Autodesk Fusion 360 part; units mm, degrees
sketch "Sketch1" plane through (0, 0, 0) normal (0, 0, 1) x (1, 0, 0)
  line L0 (0, 0) -> (385.5, 0)
  line L1 (385.5, 0) -> (385.5, 160.5)
  line L2 (385.5, 160.5) -> (0, 160.5)
  line L3 (0, 160.5) -> (0, 0)
  line L4 (10, 150.5) -> (375.5, 150.5)
  line L5 (375.5, 150.5) -> (375.5, 10)
  line L6 (375.5, 10) -> (10, 10)
  line L7 (10, 10) -> (10, 150.5)
  circle A0 centre (5, 155.5) radius 1.45
  circle A1 centre (5, 5) radius 1.45
  circle A2 centre (380.5, 5) radius 1.45
  circle A3 centre (380.5, 155.5) radius 1.45
  dimension "d1" = 160.5
  dimension "d2" = 385.5
  dimension "d3" = 10
  dimension "d4" = 10
  dimension "d5" = 10
  dimension "d6" = 10
  dimension "d7" = 2.9
  dimension "d8" = 2.9
  dimension "d9" = 2.9
  dimension "d10" = 2.9
  dimension "d11" = 5
  dimension "d12" = 5
  dimension "d13" = 5
  dimension "d14" = 5
  dimension "d15" = 5
  dimension "d16" = 5
  dimension "d17" = 5
  dimension "d18" = 5
sketch "Sketch2" plane through (0, 0, 0) normal (0, 0, 1) x (1, 0, 0)
  line L0 (0, 0) -> (385.5, 0)
  line L1 (385.5, 0) -> (385.5, 160.5)
  line L2 (385.5, 160.5) -> (0, 160.5)
  line L3 (0, 160.5) -> (0, 0)
  line L4 (375.5, 10) -> (10, 10)
  line L5 (10, 10) -> (10, 150.5)
  line L6 (10, 150.5) -> (375.5, 150.5)
  line L7 (375.5, 150.5) -> (375.5, 10)
  dimension "d21" = 160.5
  dimension "d22" = 385.5
  dimension "d23" = 10
  dimension "d24" = 10
  dimension "d25" = 365.5
  dimension "d26" = 140.5
sketch "Sketch3" plane through (0, 0, 0) normal (0, 1, 0) x (1, 0, 0)
sketch "Sketch4" plane through (0, 0, 0) normal (0, 0, 1) x (1, 0, 0)
  line L0 (0, -20) -> (385.5, -20)
  line L1 (385.5, -20) -> (385.5, -180.5)
  line L2 (385.5, -180.5) -> (0, -180.5)
  line L3 (0, -180.5) -> (0, -20)
  line L4 (375.5, -170.5) -> (10, -170.5)
  line L5 (10, -170.5) -> (10, -30)
  line L6 (10, -30) -> (375.5, -30)
  line L7 (375.5, -30) -> (375.5, -170.5)
  circle A0 centre (5, -175.5) radius 1.45
  circle A1 centre (5, -25) radius 1.45
  circle A2 centre (380.5, -25) radius 1.45
  circle A3 centre (380.5, -175.5) radius 1.45
  dimension "d29" = 160.5
  dimension "d30" = 385.5
  dimension "d31" = 10
  dimension "d32" = 10
  dimension "d33" = 10
  dimension "d34" = 10
  dimension "d35" = 2.9
  dimension "d36" = 5
  dimension "d37" = 5
  dimension "d38" = 2.9
  dimension "d39" = 5
  dimension "d40" = 5
  dimension "d41" = 2.9
  dimension "d42" = 5
  dimension "d43" = 5
  dimension "d44" = 2.9
  dimension "d45" = 5
  dimension "d46" = 5
extrude "Extrude3" add sketch "Sketch4" along normal blind 3 contours L0 L1 L2 L3 | L4 L5 L6 L7
sketch "Sketch5" plane through (0, 0, 3) normal (0, 0, 1) x (-1, 0, 0)
  circle A0 centre (-15.5, -145) radius 3.3
  circle A1 centre (-15.5, -145) radius 1.3
  circle A2 centre (-15.5, -15.5) radius 1.3
  circle A3 centre (-15.5, -15.5) radius 3.3
  circle A4 centre (-370, -15.5) radius 1.3
  circle A5 centre (-370, -15.5) radius 3.3
  circle A6 centre (-370, -145) radius 1.3
  circle A7 centre (-370, -145) radius 3.3
  line L0 (-375.5, -150.5) -> (-10, -150.5)
  line L1 (-10, -150.5) -> (-10, -10)
  line L2 (-10, -10) -> (-375.5, -10)
  line L3 (-375.5, -10) -> (-375.5, -150.5)
  dimension "d49" = 6.6
  dimension "d52" = 2.6
  dimension "d53" = 2.6
  dimension "d56" = 6.6
  dimension "d57" = 2.6
  dimension "d58" = 6.6
  dimension "d61" = 2.6
  dimension "d62" = 6.6
sketch "Sketch6" plane through (0, 0, 3) normal (0, 0, 1) x (-1, 0, 0)
  circle A0 centre (-5, 25) radius 1.45
  circle A1 centre (-5, 175.5) radius 1.45
  circle A2 centre (-380.5, 25) radius 1.45
  circle A3 centre (-380.5, 175.5) radius 1.45
  line L0 (0, 180.5) -> (-385.5, 180.5)
  line L1 (-385.5, 180.5) -> (-385.5, 20)
  line L2 (-385.5, 20) -> (0, 20)
  line L3 (0, 20) -> (0, 180.5)
sketch "Sketch7" plane through (0, 0, 0) normal (0, 0, -1) x (1, 0, 0)
  circle A0 centre (5, 25) radius 1.45
  circle A1 centre (5, 175.5) radius 1.45
  circle A2 centre (380.5, 25) radius 1.45
  circle A3 centre (380.5, 175.5) radius 1.45
  line L0 (385.5, 180.5) -> (0, 180.5)
  line L1 (0, 180.5) -> (0, 20)
  line L2 (0, 20) -> (385.5, 20)
  line L3 (385.5, 20) -> (385.5, 180.5)
  line L4 (0, 20) -> (385.5, 20)
  line L5 (385.5, 20) -> (385.5, 180.5)
  line L6 (385.5, 180.5) -> (0, 180.5)
  line L7 (0, 180.5) -> (0, 20)
  line L8 (0, 20) -> (385.5, 20)
  line L9 (385.5, 20) -> (385.5, 180.5)
  line L10 (385.5, 180.5) -> (0, 180.5)
  line L11 (0, 180.5) -> (0, 20)
  line L12 (0, 20) -> (385.5, 20)
  line L13 (385.5, 20) -> (385.5, 180.5)
  line L14 (385.5, 180.5) -> (0, 180.5)
  line L15 (0, 180.5) -> (0, 20)
  line L16 (15.5, 165) -> (370, 165)
  line L17 (370, 165) -> (370, 35.5)
  line L18 (370, 35.5) -> (15.5, 35.5)
  line L19 (15.5, 35.5) -> (15.5, 165)
  line L20 (0, 180.5) -> (385.5, 180.5)
  dimension "d68" = 15.5
  dimension "d70" = 15.5
  dimension "d71" = 15.5
  dimension "d72" = 15.5
extrude "Extrude5" cut sketch "Sketch7" against normal blind 150 contours L16 L17 L18 L19
fillet "Fillet5" radius 4 1 edges at (385.5, -180.5, 1.5)
fillet "Fillet6" radius 4 1 edges at (385.5, -20, 1.5)
fillet "Fillet7" radius 4 1 edges at (0, -180.5, 1.5)
fillet "Fillet8" radius 4 1 edges at (0, -20, 1.5)
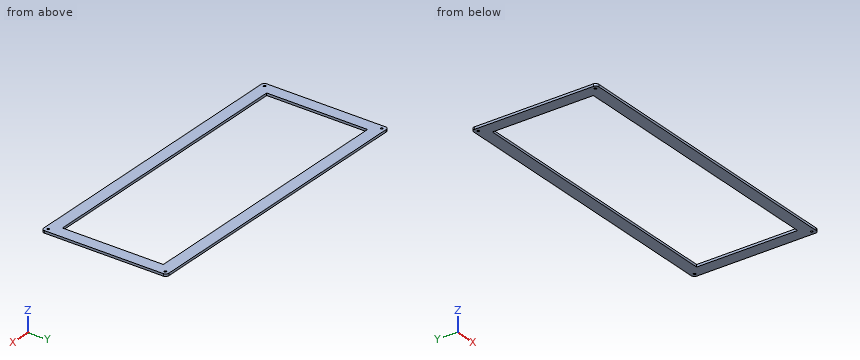
Input: part model. Units: mm. Frame: model coordinates. Give positions to 0.01 mm unless a question says otherwise; leave off trailing zeros. Order: outer loops, then holes, each group sorted by start corner. A loop starts at its lowest first (then second) coordinate and runs counter-clockwise, first axis right, second up. Notation, with made-up numbers: M 35,18.25 L 45,18.25 A9 ccw 45,25.25 Z; hole C 50.5,-26.75 d5. An arc over 180 degrees is marked long. One line per question, with ' | ' between items.
1) Section A-A on x = 85. Output: boundary loops of the cut face in (y, z), and give its area (3 significant figures).
Filled in:
outline: M -180.5,0 L -165,0 L -165,3 L -180.5,3 Z; M -35.5,0 L -20,0 L -20,3 L -35.5,3 Z | area: 93.0 mm2
2) Section B-B on y = -141. Output: boundary loops of the cut face in (x, z).
Filled in:
outline: M 0,0 L 15.5,0 L 15.5,3 L 0,3 Z; M 370,0 L 385.5,0 L 385.5,3 L 370,3 Z
3) Ray query, L1, parallel to Y at x = 380.5, z = 0.95; L2, parallel to X at y = -175.5, z = 1.6; L3, parallel to Y at x = 27, z = 2.6. Return the intervals inside material, ascending.
Filled in:
L1: y = -180.5 to -176.95, -174.05 to -26.45, -23.55 to -20 | L2: x = 0 to 3.55, 6.45 to 379.05, 381.95 to 385.5 | L3: y = -180.5 to -165, -35.5 to -20
4) Contact query for a flat-ended pin moving along its axis: P1, Ø1.5, axis at y = -96, z = 2, coming from the -X side. Output: stop coordinate, or through.
Filled in:
P1: stops at x = 0
5) Section C-C on z = 1.7. Output: boundary loops of the cut face in (x, y), and give its area (3 significant figures).
Filled in:
outline: M 0,-176.5 A4 ccw 4,-180.5 L 381.5,-180.5 A4 ccw 385.5,-176.5 L 385.5,-24 A4 ccw 381.5,-20 L 4,-20 A4 ccw 0,-24 Z; hole C 5,-175.5 d2.9; hole C 5,-25 d2.9; hole M 15.5,-165 L 370,-165 L 370,-35.5 L 15.5,-35.5 Z; hole C 380.5,-175.5 d2.9; hole C 380.5,-25 d2.9 | area: 15,900 mm2
